The model under review builds one solid part; all positions refer to its coordinate system, in mm. A direction names the side the tool comes from. Round coordinates to 2 decimals unless told otherwise and drop trailing zeros. Write each loop counter-clockwise with the first axis right and the second up, starting at its lowest first coordinate (ties: lowest second). Pieces come first, ordered by that corner, then holes. Notation, with made-up numbers: (75, 12.25) -> (103, 12.25) arc R22 ccw to (103, 28.25) -> close; hole circle Ø9 at (0.5, 28.5). An arc over 180 degrees is marked (long way). Answer in a Markdown table with one row per item. Add a question column.
```python
from build123d import *

# Parameters (mm, degrees)
F0_R     = 10
F1_DEPTH = 7.5
F2_R     = 10
F3_DEPTH = 10
F4_R     = 10
F5_DEPTH = 7.5
F6_R     = 2.5
F7_DEPTH = 25
F8_R     = 4
F9_DEPTH = 10


with BuildPart() as f1:
    # F0 (on Top) → F1 (new body)
    with BuildSketch(Plane.XY):
        Circle(F0_R)
    extrude(amount=F1_DEPTH)

    # F2 (on face) → F3 (join)
    with BuildSketch(Plane.XY.offset(7.5)):
        Circle(F2_R)
    extrude(amount=F3_DEPTH)

    # F4 (on face) → F5 (join)
    with BuildSketch(Plane.XY.offset(17.5)):
        Circle(F4_R)
    extrude(amount=F5_DEPTH)

    # F6 (on face) → F7 (cut)
    with BuildSketch(Plane.XY.offset(25)):
        Circle(F6_R)
    extrude(amount=-F7_DEPTH, mode=Mode.SUBTRACT)

    # F8 (on face) → F9 (cut)
    with BuildSketch(Plane(origin=(0, 0, 0), x_dir=(1, 0, 0), z_dir=(0, 0, -1))):
        Circle(F8_R)
    extrude(amount=-F9_DEPTH, mode=Mode.SUBTRACT)


solid = f1.part
```
1. Insertion check: pin 1 Ø3 at (x, z) = (-6, 19) entering from +Y; pin 2 Ø4 at (x, y) = (-0.5, 0.5) entering from -Z; pin 3 Ø3 at (y, z) = (2.5, 18.5) entering from -X. Each pin has a flat end and moves straight along its axis. Give the tip position at first contact, or say it passes through.
2. Add section A-A on y = 0. Write out the cut boundary in (x, z).
3. For L1, parallel to Y at x = 0, z = 19.5; L2, parallel to Z at x = -2.75, y = -2.5; L3, parallel to X at y = -2, z = 18.5, list the stretches that pass through material, from the lowest coordinate up.
4. Add section D-D on y = 8. Write out the cut boundary in (x, z).
5. Mouldability with a two-part tool opening along Y and no side actions: class faces 1 (the flat face through (-0.1, -4.3, 0)), 2 (the cylindrical face through (-2.17, -9.76, 12.32)), 3 (the cylindrical face through (-0.54, -2.44, 17.6)) as pulls with the +Y half, pulls with the -Y half, needs draft (parallel to the pull), parting line crosses it, or undercut.
6. Add section C-C on z = 2.5. Write out the cut boundary in (x, y), plus the area to 3 significant figures.
7. Tool access review of faces 4 (the cylindrical face through (-0.867, 3.905, 4.93)), 5 (the flat face through (2, -2, 25)): name each direction out of +Z, -Z, +X, -X, +Y, -Y from which nothing blocks a thin tool from reaching the whole face with its end or side.
Filled in:
| question | item | result |
|---|---|---|
| 1 | pin 1 | y = 8.93 |
| 1 | pin 2 | z = 10 |
| 1 | pin 3 | x = -9.95 |
| 2 | outline | (-10, 0) -> (-4, 0) -> (-4, 10) -> (-2.5, 10) -> (-2.5, 25) -> (-10, 25) -> close; (2.5, 10) -> (4, 10) -> (4, 0) -> (10, 0) -> (10, 25) -> (2.5, 25) -> close |
| 3 | L1 | -10 to -2.5, 2.5 to 10 |
| 3 | L2 | 10 to 25 |
| 3 | L3 | -9.8 to -1.5, 1.5 to 9.8 |
| 4 | outline | (-6, 0) -> (6, 0) -> (6, 25) -> (-6, 25) -> close |
| 5 | face 1 | needs draft |
| 5 | face 2 | parting line crosses it |
| 5 | face 3 | undercut |
| 6 | outline | circle Ø20 at (0, 0); hole circle Ø8 at (0, 0) |
| 6 | area | 264 mm² |
| 7 | face 4 | -Z |
| 7 | face 5 | +Z, +X, -X, +Y, -Y |
